```python
from build123d import *

# Parameters (mm, degrees)
SKETCH1_R                           = 2.159
BOSS_EXTRUDE1_DEPTH                 = 1.575
SKETCH2_W                           = 93.457658642
SKETCH2_H                           = 6.602
CUT_EXTRUDE1_DEPTH                  = 65.362755899
CUT_EXTRUDE2_DEPTH                  = 60.755092082
CUT_EXTRUDE3_DEPTH                  = 60.755092082
SKETCH6_R                           = 0.8382
CUT_EXTRUDE4_DEPTH                  = 2.54
SKETCH7_W                           = 65.648
SKETCH7_H                           = 12
CUT_EXTRUDE5_DEPTH                  = 59.286069146
SKETCH11_R                          = 0.412551942
ID_HOLE_DEPTH                       = 59.286069146
SKETCH12_W                          = 2.575
SKETCH12_H                          = 5
NOTCH_FOR_BPR_TOP_VIEW_DEPTH        = 59.286069146
SKETCH14_W                          = 2.575
SKETCH14_H                          = 12.502619879
NOTCH_FOR_BPL_TOP_VIEW_DEPTH        = 59.286069146
SKETCH17_W                          = 73.57
SKETCH17_H                          = 1
CREATE_LIP_FOR_M3_SPACER_HOLE_DEPTH = 1.575
SKETCH15_R                          = 1.6
HOLE_FOR_M3_SPACER_DEPTH            = 59.977069112


with BuildPart() as part:
    # Sketch1 → Boss-Extrude1 (new body)
    with BuildSketch(Plane(origin=(0, 0, 0), x_dir=(1, 0, 0), z_dir=(0, 1, 0))):
        Polygon((44.351293299, -40.014412246), (37.136293299, -40.014412246), (37.136293299, -46.615946892), (29.968293307, -46.615946892), (-30.083706693, -46.615946892), (-36.433706701, -46.615946892), (-36.433706701, -40.014412246), (-43.648706701, -40.014412246), (-43.648706701, -30.885946892), (-43.648706701, -29.647946892), (-42.378706693, -29.615946892), (-32.472706701, -29.647946892), (-32.472706701, -10.370428445), (-12.155556701, -10.370428445), (-12.155556701, -34.615947016), (-11.557706701, -34.615947016), (12.260293299, -34.615947016), (12.858143299, -34.615947016), (12.858143299, -10.370428445), (33.175293299, -10.370428445), (33.175293299, -12.929386892), (33.175293299, -29.647946892), (38.746293307, -29.615946892), (42.351293307, -29.615946892), (44.351293299, -29.615946892), (44.351293299, -31.651946892), align=None)
        with Locations(Location((-19.648556701, -28.76738335, 0), (0, 0, 270))):
            Circle(SKETCH1_R, mode=Mode.SUBTRACT)
        with Locations(Location((-19.648556701, -20.63938335, 0), (0, 0, 270))):
            Circle(SKETCH1_R, mode=Mode.SUBTRACT)
        with Locations(Location((20.351397299, -20.63938335, 0), (0, 0, 270))):
            Circle(SKETCH1_R, mode=Mode.SUBTRACT)
        with Locations(Location((20.351397299, -28.76738335, 0), (0, 0, 270))):
            Circle(SKETCH1_R, mode=Mode.SUBTRACT)
    extrude(amount=BOSS_EXTRUDE1_DEPTH)

    # Sketch2 → Cut-Extrude1 (cut, through all)
    with BuildSketch(Plane.XZ):
        with Locations((-2.377536022, 43.315412246)):
            Rectangle(SKETCH2_W, SKETCH2_H)
    extrude(amount=-CUT_EXTRUDE1_DEPTH, mode=Mode.SUBTRACT)

    # Sketch3 → Cut-Extrude2 (cut, through all)
    with BuildSketch(Plane.XZ):
        Polygon((-41.504650493, 40.014412246), (-41.504650493, 29.618770413), (-34.629650483, 29.640979175), (-34.629650483, 8.976090323), (-48.128778183, 8.976090323), (-48.128778183, 40.014412246), align=None)
    extrude(amount=-CUT_EXTRUDE2_DEPTH, mode=Mode.SUBTRACT)

    # Sketch4 → Cut-Extrude3 (cut, through all)
    with BuildSketch(Plane.XZ):
        Polygon((42.351293299, 40.014412246), (42.351293299, 32.420104455), (42.351293299, 29.615946892), (35.476293307, 29.615946892), (35.476293307, 10.370428445), (54.710892309, 10.370428445), (54.710892309, 40.014412246), align=None)
    extrude(amount=-CUT_EXTRUDE3_DEPTH, mode=Mode.SUBTRACT)

    # Sketch6 → Cut-Extrude4 (cut)
    with BuildSketch(Plane(origin=(0, 0, 0), x_dir=(-1, 0, 0), z_dir=(0, -1, 0))):
        with Locations(Location((27.141556701, -35.947946892, 0), (0, 0, 90))):
            Circle(SKETCH6_R)
        with Locations(Location((27.141556701, -25.025946892, 0), (0, 0, 90))):
            Circle(SKETCH6_R)
        with Locations(Location((14.695556701, -25.025946892, 0), (0, 0, 90))):
            Circle(SKETCH6_R)
        with Locations(Location((-15.398143299, -25.025946892, 0), (0, 0, 90))):
            Circle(SKETCH6_R)
        with Locations(Location((-27.844397299, -25.025946892, 0), (0, 0, 90))):
            Circle(SKETCH6_R)
        with Locations(Location((-27.844397299, -35.947946892, 0), (0, 0, 90))):
            Circle(SKETCH6_R)
    extrude(amount=-CUT_EXTRUDE4_DEPTH, mode=Mode.SUBTRACT)

    # Sketch7 → Cut-Extrude5 (cut, through all)
    with BuildSketch(Plane.XZ):
        with Locations((0.351293299, 16.370428445)):
            Rectangle(SKETCH7_W, SKETCH7_H)
    extrude(amount=-CUT_EXTRUDE5_DEPTH, mode=Mode.SUBTRACT)

    # Sketch11 → ID HOLE (cut, through all)
    with BuildSketch(Plane(origin=(0, 1.575, 0), x_dir=(1, 0, 0), z_dir=(0, 1, 0))):
        with Locations(Location((-39.304798754, -30.495020326, 0), (0, 0, 270))):
            Circle(SKETCH11_R)
    extrude(amount=-ID_HOLE_DEPTH, mode=Mode.SUBTRACT)

    # Sketch12 → Notch for BPR (TOP VIEW) (cut, through all)
    with BuildSketch(Plane(origin=(0, 0, 0), x_dir=(-1, 0, 0), z_dir=(0, -1, 0))):
        with Locations((35.201150493, -32.134973926)):
            Rectangle(SKETCH12_W, SKETCH12_H)
    extrude(amount=-NOTCH_FOR_BPR_TOP_VIEW_DEPTH, mode=Mode.SUBTRACT)

    # Sketch14 → Notch for BPL (TOP VIEW) (cut, through all)
    with BuildSketch(Plane(origin=(0, 0, 0), x_dir=(-1, 0, 0), z_dir=(0, -1, 0))):
        with Locations((-36.253849507, -28.621738385)):
            Rectangle(SKETCH14_W, SKETCH14_H)
    extrude(amount=-NOTCH_FOR_BPL_TOP_VIEW_DEPTH, mode=Mode.SUBTRACT)

    # Sketch17 → Create Lip for M3 Spacer Hole (add)
    with BuildSketch(Plane.XZ):
        with Locations((0.351293299, 40.514412246)):
            Rectangle(SKETCH17_W, SKETCH17_H)
    extrude(amount=-CREATE_LIP_FOR_M3_SPACER_HOLE_DEPTH)

    # Sketch15 → HOLE for M3 Spacer (cut, through all)
    with BuildSketch(Plane.XZ):
        with Locations(Location((-0.006565304, 37.835831124, 0), (0, 0, 270))):
            Circle(SKETCH15_R)
        with Locations(Location((-33.628715371, 37.835831124, 0), (0, 0, 270))):
            Circle(SKETCH15_R)
        with Locations(Location((34.851293299, 37.835831124, 0), (0, 0, 270))):
            Circle(SKETCH15_R)
    extrude(amount=-HOLE_FOR_M3_SPACER_DEPTH, mode=Mode.SUBTRACT)


solid = part.part
```
For this review, take the finished solid that the model builds, in its own axes (mm). A direction names the side the tool comes from. Coordinates: 2 decimals unless noted, no trailing zeros. Write each loop counter-clockwise with the first axis right and the second up, starting at its lowest first coordinate (ties: lowest second). Pieces come first, ordered by that corner, then holes. Notation, with made-up numbers: (10, -20) -> (25, -20) arc R14 ccw to (25, 4) -> close; hole circle Ø7 at (-2, -27). An arc over 180 degrees is marked (long way). Put each result on its own line as item: value.
Q1. Take a section at C-C, the plane z = 28. State the section outline as (x, y) points (3 decimals), then the cut area to 3 significant figures.
From the geometry:
outline: (-32.473, 0) -> (-21.667, 0) -> (-21.667, 1.575) -> (-32.473, 1.575) -> close; (-17.631, 0) -> (-12.156, 0) -> (-12.156, 1.575) -> (-17.631, 1.575) -> close; (12.858, 0) -> (18.333, 0) -> (18.333, 1.575) -> (12.858, 1.575) -> close; (22.369, 0) -> (33.175, 0) -> (33.175, 1.575) -> (22.369, 1.575) -> close
area: 51.3 mm2
Q2. The part is to be moulded in two halves that separate along X. For faces 4 (the flat face through (-27, 1, 22.37)), 5 (the flat face through (-32.473, 1, 26)), 6 (the flat face through (12.858, 1, 29)), say which applies: +X half, -X half, draft (parallel to the pull), parting line (faces both ways), or undercut.
From the geometry:
face 4: draft
face 5: -X half
face 6: undercut
Q3. Take a section at D-D, the plane y = 1.3. Count the separate pieces of the cut face and the enclosed holes in it, then the cut area to 3 significant figures.
From the geometry:
separate pieces: 1
enclosed holes: 12
area: 1,020 mm2
Q4. Tool access review of faces 1 (the cylindrical face through (33.29, 0.78, 38.18)), 2 (the flat face through (-36.489, 1, 32)), 3 (the flat face through (41, 1, 29.616)): name each direction out of +Z, -Z, +X, -X, +Y, -Y from which nothing blocks a thin tool from reaching the whole face with its end or side.
From the geometry:
face 1: +Y, -Y
face 2: -Z, +Y, -Y
face 3: -Z, +X, +Y, -Y
Q5. Take a section at B-B, the plane x = 9. State the section outline as (y, z) points (3 decimals), then the cut area to 3 significant figures.
From the geometry:
outline: (0, 34.616) -> (1.575, 34.616) -> (1.575, 41.014) -> (0, 41.014) -> close
area: 10.1 mm2
Q6. Take a section at A-A, the plane z = 33.25. State the section outline as (x, y) points (3 decimals), then the cut area to 3 significant figures.
From the geometry:
outline: (-41.505, 0) -> (-36.489, 0) -> (-36.489, 1.575) -> (-41.505, 1.575) -> close; (-33.914, 0) -> (-12.156, 0) -> (-12.156, 1.575) -> (-33.914, 1.575) -> close; (12.858, 0) -> (34.966, 0) -> (34.966, 1.575) -> (12.858, 1.575) -> close; (37.541, 0) -> (42.351, 0) -> (42.351, 1.575) -> (37.541, 1.575) -> close
area: 84.6 mm2
Q7. Clearance check with flat-ended pins moving along their axes: pin 1 Ø4 at (x, z) = (34.85, 37.84) entering from -Y; pin 2 Ø0.8 at (x, y) = (38.5, 1) entering from +Z; pin 3 Ø0.8 at (y, z) = (0.5, 28) entering from -X; pin 4 Ø0.8 at (y, z) = (0.5, 40.5) entering from +X. State where each tip first meets the part, or that it passes through.
From the geometry:
pin 1: stops at y = 0
pin 2: stops at z = 40.01
pin 3: stops at x = -32.47
pin 4: stops at x = 37.14
Q8. Wall thickness on L1, parallel to X at y = 0.75, z = 34; L2, parallel to X at y = 0.65, z = 37.75; L3, parallel to X at y = 0.5, z = 35.5: over which ranges is each line inside the solid? List them lowest first.
From the geometry:
L1: x = -41.5 to -36.49, -33.91 to -12.16, 12.86 to 34.97, 37.54 to 42.35
L2: x = -41.5 to -35.23, -32.03 to -1.6, 1.59 to 33.25, 36.45 to 42.35
L3: x = -41.5 to -27.85, -26.43 to 27.14, 28.55 to 42.35
